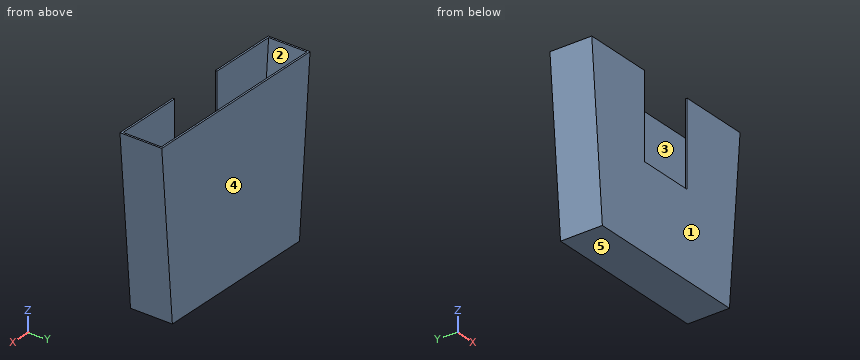
```python
from build123d import *

# Parameters (mm, degrees)
F1_DEPTH = 76.2
F2_T     = -3.175
F3_W     = 50.8
F3_H     = 76.2
F4_DEPTH = 25.4


with BuildPart() as f1:
    # F0 (on Front) → F1 (new body)
    with BuildSketch(Plane.XZ):
        Polygon((177.8, 0), (0, 0), (-177.8, 0), (-152.4, -304.8), (0, -304.8), (152.4, -304.8), align=None)
    extrude(amount=F1_DEPTH)

    # F2
    f2_openings = [f1.faces().sort_by_distance(p)[0] for p in [
        (0, -38.1, 0),
    ]]
    offset(amount=F2_T, openings=f2_openings)

    # F3 (on face) → F4 (cut)
    with BuildSketch(Plane.XZ.offset(76.2)):
        with Locations((-25.4, -114.3)):
            Rectangle(F3_W, F3_H)
        with Locations((-25.4, -38.1)):
            Rectangle(F3_W, F3_H)
        with Locations((25.4, -38.1)):
            Rectangle(F3_W, F3_H)
        with Locations((25.4, -114.3)):
            Rectangle(F3_W, F3_H)
    extrude(amount=-F4_DEPTH, mode=Mode.SUBTRACT)


solid = f1.part
```
The listing builds one solid part. Answer for the finished solid, in the listing's coordinates (mm). Face numbers are marked on the shaded views. A direction names the side the tool comes from. Coordinates: 2 decimals unless noted, no trailing zeros. Loops run counter-clockwise (first coordinate to the right, second up) from the corner with the lowest first, then second, coordinate; pieces in that order, holes last. Notation, with made-up numbers: (30, -22.75) -> (73, -22.75) arc R25 ccw to (73, 5.25) -> close; hole circle Ø10 at (4, 75). An arc over 180 degrees is marked (long way). Use one line per item in the form item = value. Start each with the question number.
Item 1: The mould has two halves that part along Y. Classify the marked faces 3, 4 and 5: released by +Y, released by -Y, zero draft, split by the parting line, or undercut.
Item 2: The part is cut by section D-D on z = -35.5. Determine the outline of the cut face in (x, y) (3 decimals).
Item 3: The part is cut by section C-C on y = -26.5. Determine the outline of the cut face in (x, z) (3 decimals), then the cut area to 3 significant figures.
Item 4: The part is cut by section A-A on x = 4.5. Determine the outline of the cut face in (y, z) (3 decimals).
Item 5: A tool of negligible diameter and unlimited length cuts with its end or side. For the marked faces 1 and 2, from which of +Z, -Z, +X, -X, +Y, -Y can it reach the whole face along a straight path? Write none if from no direction.
Item 6: Flat-ended cylindrical pins translate along their axes: pin 1 Ø2.5 at (x, y) = (-6, -74) entering from +Z; pin 2 Ø1.5 at (x, y) = (-9.5, -61.5) entering from +Z (3 decimals); pin 3 Ø1 at (y, z) = (-74.5, -111.5) entering from -X. Find the tip coordinate at first contact, or state that the pin passes through.
Item 7: Consider L1, parallel to Y at x = -49, z = -154 (3 decimals); L2, parallel to Z at x = -147, y = -9 (3 decimals); L3, parallel to X at y = -4.5, z = -56.5. Determine where each line is inside the solid, lowest interval first. Write a range as [from, to].
Item 8: The part is cut by section B-B on z = -257. Determine the outline of the cut face in (x, y) (3 decimals).
Answer key:
q1.face_3 = undercut
q1.face_4 = released by +Y
q1.face_5 = zero draft
q2.outline = (-174.842, -76.2) -> (-50.8, -76.2) -> (-50.8, -73.025) -> (-171.656, -73.025) -> (-171.656, -3.175) -> (171.656, -3.175) -> (171.656, -73.025) -> (50.8, -73.025) -> (50.8, -76.2) -> (174.842, -76.2) -> (174.842, 0) -> (-174.842, 0) -> close
q3.outline = (-177.8, 0) -> (-152.4, -304.8) -> (152.4, -304.8) -> (177.8, 0) -> (174.614, 0) -> (149.479, -301.625) -> (-149.479, -301.625) -> (-174.614, 0) -> close
q3.area = 2,890 mm2
q4.outline = (-76.2, -304.8) -> (0, -304.8) -> (0, 0) -> (-3.175, 0) -> (-3.175, -301.625) -> (-73.025, -301.625) -> (-73.025, -152.4) -> (-76.2, -152.4) -> close
q5.face_1 = +Z, -Z, +X, -X, -Y
q5.face_2 = +Z
q6.pin_1 = -152.4
q6.pin_2 = -301.625
q6.pin_3 = -168.55
q7.L1 = [-76.2, -73.025], [-3.175, 0]
q7.L2 = [-304.8, -301.625]
q7.L3 = [-173.09, -169.91], [169.91, 173.09]
q8.outline = (-156.383, -76.2) -> (156.383, -76.2) -> (156.383, 0) -> (-156.383, 0) -> close; hole (-153.197, -73.025) -> (153.197, -73.025) -> (153.197, -3.175) -> (-153.197, -3.175) -> close
